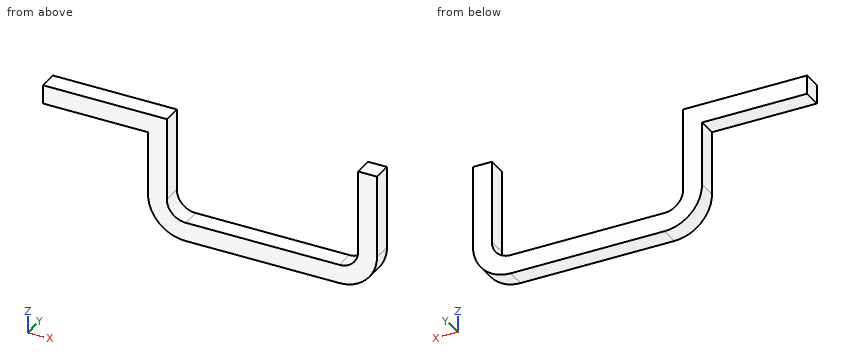
from build123d import *

# Parameters (mm, degrees)
BOSS_EXTRUDE1_DEPTH = 10


with BuildPart() as part:
    # Sketch1 → Boss-Extrude1 (new body)
    with BuildSketch(Plane(origin=(0, 0, 0), x_dir=(1, 0, 0), z_dir=(0, 1, 0))):
        with BuildLine():
            Line((0, 0), (29.149551568, 0))
            Line((29.149551568, 0), (29.149551568, 43.975))
            ThreePointArc((29.149551568, 43.975), (32.078483756, 51.046067812), (39.149551568, 53.975))
            Line((39.149551568, 53.975), (120.749551568, 53.975))
            ThreePointArc((120.749551568, 53.975), (127.82061938, 51.046067812), (130.749551568, 43.975))
            Line((130.749551568, 43.975), (130.749551568, 0))
            Line((130.749551568, 0), (140.749551568, 0))
            Line((140.749551568, 0), (140.749551568, 43.975))
            ThreePointArc((140.749551568, 43.975), (134.891687192, 58.117135624), (120.749551568, 63.975))
            Line((120.749551568, 63.975), (39.149551568, 63.975))
            ThreePointArc((39.149551568, 63.975), (25.007415944, 58.117135624), (19.149551568, 43.975))
            Line((19.149551568, 43.975), (19.149551568, 10))
            Line((19.149551568, 10), (0, 10))
            Line((0, 10), (-36.600725287, 10))
            Line((-36.600725287, 10), (-36.600725287, 0))
            Line((-36.600725287, 0), (0, 0))
        make_face()
    extrude(amount=BOSS_EXTRUDE1_DEPTH)


solid = part.part
Geometry check sheet. Reference: the model listing, model coordinates, mm. Coordinates: 2 decimals unless noted, no trailing zeros. Order: outer loops, then holes, each group sorted by start corner. A loop starts at its lowest first (then second) coordinate and runs counter-clockwise, first axis right, second up. Notation, with made-up numbers: (59, -26) - (75, -26) arc R14 cw to (75, -12) - close; hole circle Ø9 at (23, -31). An arc over 180 degrees is marked (long way). Answer in a Markdown table with one row per item. Add a question column.
1) Cross-section at B-B, the plane y = 5.5. Record the cut outline in (x, z) (3 decimals), then the cut area to 3 significant figures.
2) Material ranges on line 1 along X through (y, z) = (4.25, -13); line 2 along X through (y, z) = (5.5, -3.5); line 3 along Z through (x, y) = (93.5, 2.75) (3 decimals), recorded low to high. Write a range as [from, to].
3) Cross-section at C-C, the plane z = -49. Record the cut outline in (x, y).
4) Cross-section at A-A, the plane z = -12.5. Record the cut outline in (x, y), then the cut area to 3 significant figures.
5) Gauge pin test, flat ends, axial feed: P1, Ø5, axis at y = 7, z = -29, coming from the -X side; P2, Ø5, axis at x = 79.5, y = 4, coming from the +Z side (3 decimals). Record the tip position at first contact, or that the pin passes through.
6) Cross-section at D-D, the plane x = 13.5. Record the cut outline in (y, z).
Check result:
| question | item | result |
|---|---|---|
| 1 | outline | (-36.601, -10) - (19.15, -10) - (19.15, -43.975) arc R20 ccw to (39.15, -63.975) - (120.75, -63.975) arc R20 ccw to (140.75, -43.975) - (140.75, 0) - (130.75, 0) - (130.75, -43.975) arc R10 cw to (120.75, -53.975) - (39.15, -53.975) arc R10 cw to (29.15, -43.975) - (29.15, 0) - (-36.601, 0) - close |
| 1 | area | 2,720 mm² |
| 2 | line 1 | x = [19.15, 29.15], [130.75, 140.75] |
| 2 | line 2 | x = [-36.6, 29.15], [130.75, 140.75] |
| 2 | line 3 | z = [-63.975, -53.975] |
| 3 | outline | (19.79, 0) - (30.5, 0) - (30.5, 10) - (19.79, 10) - close; (129.4, 0) - (140.11, 0) - (140.11, 10) - (129.4, 10) - close |
| 4 | outline | (19.15, 0) - (29.15, 0) - (29.15, 10) - (19.15, 10) - close; (130.75, 0) - (140.75, 0) - (140.75, 10) - (130.75, 10) - close |
| 4 | area | 200 mm² |
| 5 | P1 | stops at x = 19.15 |
| 5 | P2 | stops at z = -53.975 |
| 6 | outline | (0, -10) - (10, -10) - (10, 0) - (0, 0) - close |
